Could you check a few things on this model? Use its own coordinates, in mm. Face numbers are marked on the shaded views. A direction names the side the tool comes from. Give positions to 0.01 mm unless a question says otherwise; leave off trailing zeros. Loops run counter-clockwise (first coordinate to the right, second up) from the corner with the lowest first, then second, coordinate; pieces in that order, holes last. Notation, with made-up numbers: (40, 57.5) - (63, 57.5) arc R14 ccw to (63, 75.5) - close; hole circle Ø3 at (54, -39). An arc over 180 degrees is marked (long way). One line per item, written item: value. Start each with the question number.
Q1. If I drill on line 1 (Y direction, x = -2, z = 3.5); line 2 (Y direction, x = 12, z = 5.75); line 3 (X direction, y = 6.5, z = 2.5), over which ranges is the centre line in solid material (lowest first)? Write a range as from..to.
Q2. If we mould it in two halves opening along Y, with no side actions, what happens to the marked faces 1, 2 and 3? For each: released by +Y, released by -Y, zero draft, split by the parting line, or undercut.
Q3. I'm going to push flat-ended pins straight in: P1, Ø13, axis at x = 11.88, y = 7.82, coming from the +Z side; P2, Ø3, axis at x = 24.5, z = 3, coming from the +Y side; P3, Ø2, axis at y = 21, z = 3, coming from the -X side; P4, Ø3, axis at y = 24.5, z = 3, coming from the -X side. Where does each tip first touch, or does it pass through?
Q4. I want a section at C-C (z = 8.25). Please give me the cut outline in (x, y), then the cut area to 3 significant figures.
Q5. For the marked faces 4 and 5, which set-ups out of +Z, -Z, +X, -X, +Y, -Y let a thin tool reach every point of the face, with its end or its side?
Q6. I want a section at D-D (y = 5.5). Please give me the cut outline in (x, z).
Q7. I want a section at A-A (y = 26). Please give me the cut outline in (x, z).
Q8. I want a section at B-B (x = 9). Please give me the cut outline in (y, z).
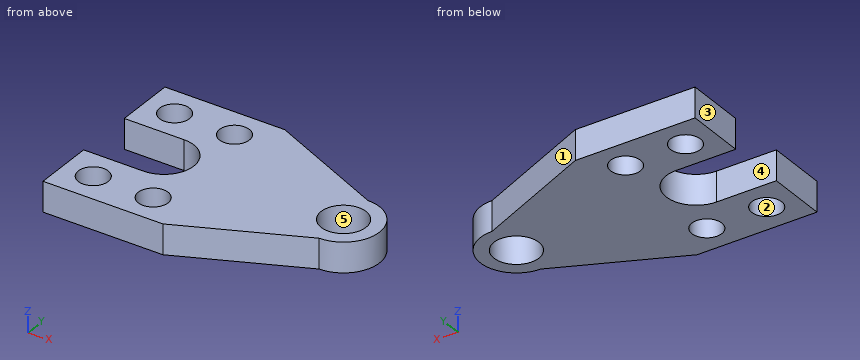
Autodesk Inventor part; units mm, degrees
ref_plane "YZ Plane" through (0, 0, 0) normal (1, 0, 0) x (0, 1, 0)
ref_plane "XZ Plane" through (0, 0, 0) normal (0, 1, 0) x (-1, 0, 0)
ref_plane "XY Plane" through (0, 0, 0) normal (0, 0, 1) x (1, 0, 0)
sketch "Эскиз1" plane through (0, 0, 0) normal (0, 0, 1) x (1, 0, 0)
  line L0 (-18.1191, -2.1753) -> (21.8809, -2.1753)
  line L1 (-18.1191, -2.1753) -> (-18.1191, 17.8247)
  line L2 (-18.1191, 17.8247) -> (1.8809, 17.8247)
  line L3 (-18.1191, 57.8247) -> (-18.1191, 37.8247)
  line L4 (-18.1191, 37.8247) -> (1.8809, 37.8247)
  line L5 (-18.1191, 57.8247) -> (21.8809, 57.8247)
  arc A0 (1.8809, 17.8247) -> (1.8809, 37.8247) centre (1.8809, 27.8247) ccw
  circle A1 centre (61.8809, 27.8247) radius 7.5
  line L6 (21.8809, 57.8247) -> (61.8809, 39.8247)
  line L7 (21.8809, -2.1753) -> (61.8809, 15.8247)
  arc A2 (61.8809, 15.8247) -> (61.8809, 39.8247) centre (61.8809, 27.8247) ccw
  circle A3 centre (-8.1191, 47.8247) radius 5
  circle A4 centre (-8.1191, 7.8247) radius 5
  circle A5 centre (11.8809, 47.8247) radius 5
  circle A6 centre (11.8809, 7.8247) radius 5
  point P0 (0, 0)
  dimension "j" = 40
  dimension "p" = 20
  dimension "g1" = 20
  dimension "d" = 60
  dimension "p1" = 20
  dimension "R1" = 15
  dimension "t" = 12
  dimension "r" = 10
  dimension "u" = 20
  dimension "a" = 80
  dimension "f1" = 10
sketch "Эскиз2" plane through (0, 0, 0) normal (0, 0, 1) x (1, 0, 0)
  point P0 (0, 0)
sketch "Эскиз3" plane through (0, 0, 0) normal (0, 0, 1) x (1, 0, 0)
  point P0 (0, 0)
extrude "Выдавливание1" add sketch "Эскиз1" along normal blind 10
properties part number "Model"
Worked answers:
1. line 1: y = -2.18..17.82, 37.82..57.82
1. line 2: y = -2.18..2.83, 12.82..42.83, 52.82..57.82
1. line 3: x = -18.12..-12.94, -3.3..7.06, 16.7..41.16
2. face 1: released by +Y
2. face 2: undercut
2. face 3: zero draft
3. P1: stops at z = 10
3. P2: stops at y = 57.32
3. P3: stops at x = 8.11
3. P4: stops at x = 10.64
4. outline: (-18.12, -2.18) - (21.88, -2.18) - (61.88, 15.82) arc R12 ccw to (61.88, 39.82) - (21.88, 57.82) - (-18.12, 57.82) - (-18.12, 37.82) - (1.88, 37.82) arc R10 cw to (1.88, 17.82) - (-18.12, 17.82) - close; hole circle Ø10 at (-8.12, 7.82); hole circle Ø10 at (-8.12, 47.82); hole circle Ø10 at (11.88, 7.82); hole circle Ø10 at (11.88, 47.82); hole circle Ø15 at (61.88, 27.82)
4. area: 3,260 mm²
5. face 4: +Z, -Z, -X
5. face 5: +Z, -Z
6. outline: (-18.12, 0) - (-12.55, 0) - (-12.55, 10) - (-18.12, 10) - close; (-3.69, 0) - (7.45, 0) - (7.45, 10) - (-3.69, 10) - close; (16.31, 0) - (38.94, 0) - (38.94, 10) - (16.31, 10) - close
7. outline: (11.71, 0) - (54.61, 0) - (54.61, 10) - (11.71, 10) - close; (69.16, 0) - (73.74, 0) - (73.74, 10) - (69.16, 10) - close
8. outline: (-2.18, 0) - (3.74, 0) - (3.74, 10) - (-2.18, 10) - close; (11.91, 0) - (20.8, 0) - (20.8, 10) - (11.91, 10) - close; (34.85, 0) - (43.74, 0) - (43.74, 10) - (34.85, 10) - close; (51.91, 0) - (57.82, 0) - (57.82, 10) - (51.91, 10) - close
